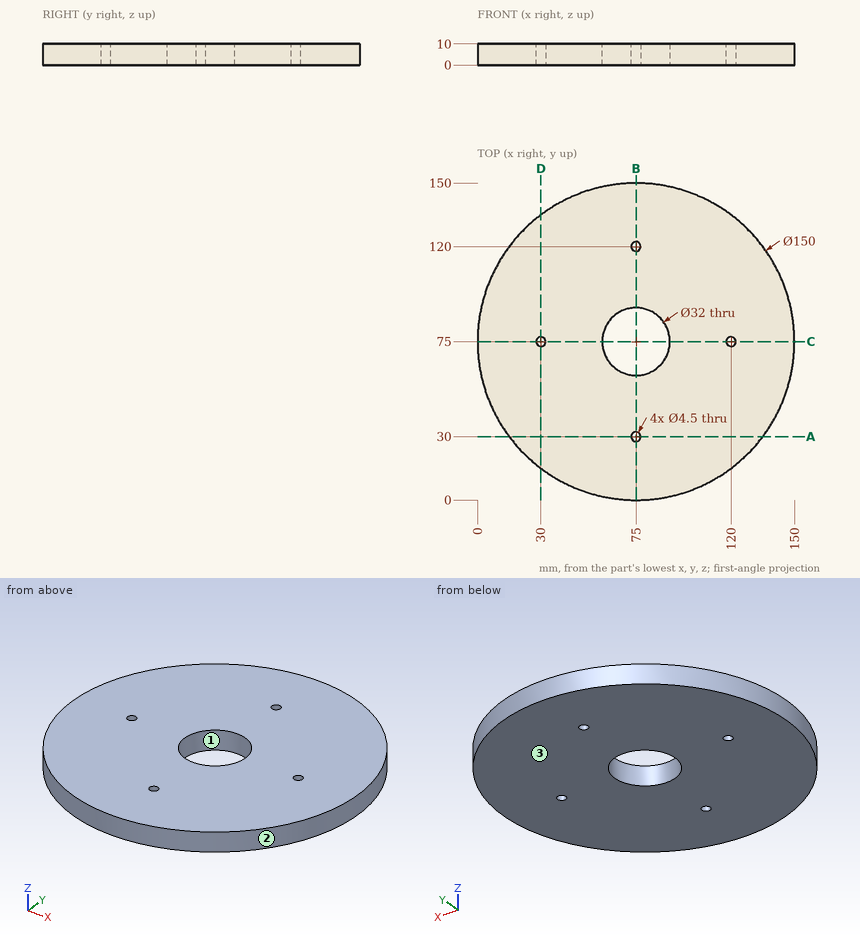
Here's the drawing with two shaded views (mm, measured from the low corner). I have some questions. Coordinates: 2 decimals unless noted, no trailing zeros. Order: outer loops, then holes, each group sorted by start corner. A loop starts at its lowest first (then second) coordinate and runs counter-clockwise, first axis right, second up. Notation, with made-up numbers: (17, -23.5) - (26, -23.5) arc R25 cw to (26, 1.5) - close; hole circle Ø3 at (39, 76.5). An arc over 180 degrees is marked (long way). Use CSV: the item, a comma, the result in double quotes. Start each with the question number.
1. Please list where these lines run through material, in increasing order: line 1 (Y direction, x = 75, z = 2.5); line 2 (Y direction, x = 30, z = 7); line 3 (X direction, y = 82, z = 9.75). Write a range as from..to.
2. Suppose I cut it at A-A on y = 30. List the corners of the cut face in (x, z) for me, then the cut area to 4 significant figures.
3. Suppose I cut it at B-B on x = 75. List the corners of the cut face in (y, z) for me.
4. I'm going to push flat-ended pins straight in: pin 1 (2 mm diameter, centred on y = 48, z = 2.5, fed in from -X); pin 2 (1 mm diameter, centred on y = 95, z = 5.5, fed in from +X); pin 3 (5 mm diameter, centred on x = 25.5, z = 7, fed in from +Y). Where does each tip first touch, or does it pass through?
5. If we mould it in two halves opening along X, with no side actions, what happens to the marked faces 1, 2 and 3? For each: +X half, -X half, draft (parallel to the pull), parting line (faces both ways), or undercut.
Output:
1,line 1,"y = 0..27.75, 32.25..59, 91..117.75, 122.25..150"
1,line 2,"y = 15..72.75, 77.25..135"
1,line 3,"x = 0.33..60.61, 89.39..149.67"
2,outline,"(15, 0) - (72.75, 0) - (72.75, 10) - (15, 10) - close; (77.25, 0) - (135, 0) - (135, 10) - (77.25, 10) - close"
2,area,"1,155 mm2"
3,outline,"(0, 0) - (27.75, 0) - (27.75, 10) - (0, 10) - close; (32.25, 0) - (59, 0) - (59, 10) - (32.25, 10) - close; (91, 0) - (117.75, 0) - (117.75, 10) - (91, 10) - close; (122.25, 0) - (150, 0) - (150, 10) - (122.25, 10) - close"
4,pin 1,"stops at x = 4.65"
4,pin 2,"stops at x = 147.42"
4,pin 3,"stops at y = 133.45"
5,face 1,"undercut"
5,face 2,"parting line"
5,face 3,"draft"
